For this review, use the dimensioned drawing (mm, ordinates from the lowest corner) and the shaded views. Coordinates: 2 decimals unless noted, no trailing zeros. Loops run counter-clockwise (first coordinate to the right, second up) from the corner with the lowest first, then second, coordinate; pieces in that order, holes last.
1. Mouldability with a two-part tool opening along Y and no side actions: class the marked faces 1, 2 and 3 as pulls with the +Y half, pulls with the -Y half, needs draft (parallel to the pull), parting line crosses it, or undercut.
2. To check wall thickness, follow probe 1 along Y at (x, z) = (14, 22); probe 2 along Y at (x, z) = (15, 20); probe 3 along Z at (x, y) = (15.5, 3). State the ranges of each line that lie inside material, in increasing order.
3. Take a section at D-D, the plane z = 30.5. State the section outline as (x, y) points, then the cut area to 3 significant figures.
4. Take a section at C-C, the plane z = 21. State the section outline as (x, y) points.
5. Take a section at A-A, the plane y = 14. State the section outline as (x, z) points, then the cut area to 3 significant figures.
6. Clearance check with flat-ended pins moving along their axes: P1, Ø8, axis at y = 6, z = 23, coming from the -X side; P2, Ø2, axis at x = 18.5, z = 14.5, coming from the +Y side; P3, Ø7, axis at x = 14, y = 14, coming from the +Z side. State where each tip first meets the part, or that it passes through.
7. Take a section at B-B, the plane x = 14. State the section outline as (y, z) points, then the cut area to 3 significant figures.
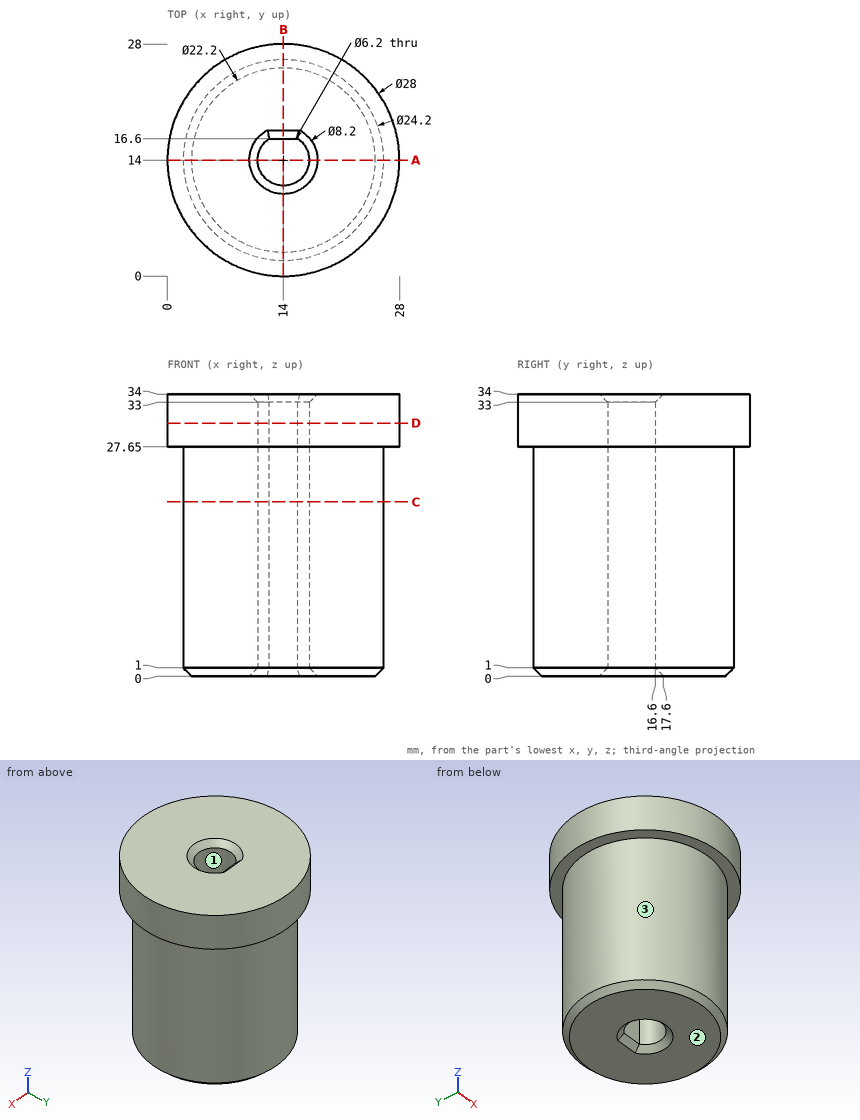
Results list:
1. face 1: undercut
1. face 2: needs draft
1. face 3: parting line crosses it
2. probe 1: y = 1.9 to 10.9, 16.6 to 26.1
2. probe 2: y = 1.94 to 11.07, 16.6 to 26.06
2. probe 3: z = 0 to 34
3. outline: circle Ø28 at (14, 14); hole (12.31, 16.6) arc R3.1 ccw (long way) to (15.69, 16.6) - close
3. area: 587 mm2
4. outline: circle Ø24.2 at (14, 14); hole (12.31, 16.6) arc R3.1 ccw (long way) to (15.69, 16.6) - close
5. outline: (0, 27.65) - (1.9, 27.65) - (1.9, 1) - (2.9, 0) - (9.9, 0) - (10.9, 1) - (10.9, 33) - (9.9, 34) - (0, 34) - close; (17.1, 1) - (18.1, 0) - (25.1, 0) - (26.1, 1) - (26.1, 27.65) - (28, 27.65) - (28, 34) - (18.1, 34) - (17.1, 33) - close
5. area: 633 mm2
6. P1: stops at x = 2.58
6. P2: stops at y = 25.58
6. P3: stops at z = 33.9
7. outline: (0, 27.65) - (1.9, 27.65) - (1.9, 1) - (2.9, 0) - (9.9, 0) - (10.9, 1) - (10.9, 33) - (9.9, 34) - (0, 34) - close; (16.6, 1) - (17.6, 0) - (25.1, 0) - (26.1, 1) - (26.1, 27.65) - (28, 27.65) - (28, 34) - (17.6, 34) - (16.6, 33) - close
7. area: 650 mm2
